Answer from the drawing. Dimensions are ordinates in mm from the lowest x, y and z of the part. A direction names the side the tool comes from. Give positions to 0.01 mm unless a question says otherwise; leave off trailing zeros. Order: outer loops, then holes, each group sorted by start corner. A loop starts at its lowest first (then second) coordinate and runs counter-clockwise, first axis right, second up.
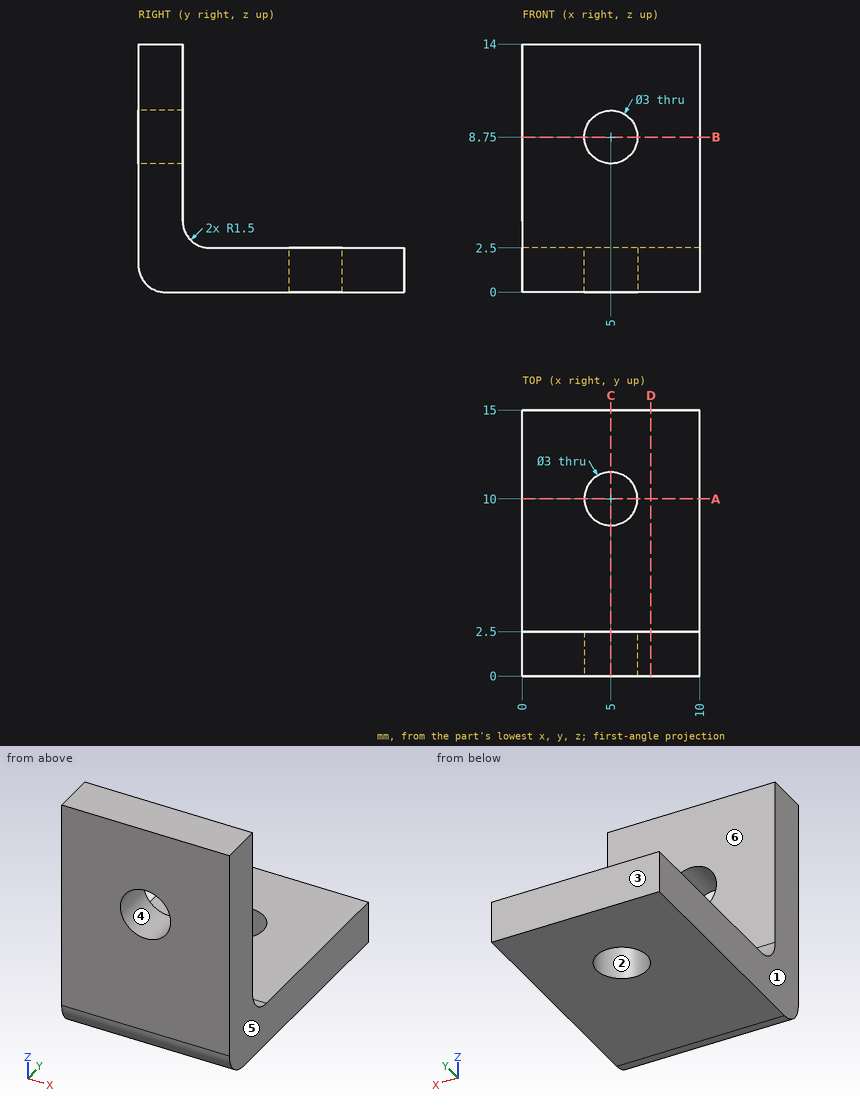
1) For a pull along X with two mould halves and no side action, classify the marked faces 1, 2, 3 and 4 as released by +X, released by -X, zero draft, split by the parting line, or undercut.
Final values:
face 1: released by -X
face 2: undercut
face 3: zero draft
face 4: undercut
2) A tool of negligible diameter and unlimited length cuts with its end or side. For the marked faces 5 and 6, from which of +Z, -Z, +X, -X, +Y, -Y can it reach the whole face along a straight path? Write none if from no direction.
Final values:
face 5: +Z, -Z, +X, +Y, -Y
face 6: +Z, +X, -X, +Y
3) The part is cut by section A-A on y = 10. Determine the outline of the cut face in (x, z).
Final values:
outline: (0, 0) - (3.5, 0) - (3.5, 2.5) - (0, 2.5) - close; (6.5, 0) - (10, 0) - (10, 2.5) - (6.5, 2.5) - close
4) The part is cut by section D-D on x = 7.25. Determine the outline of the cut face in (y, z), and give its area (4 significant figures).
Final values:
outline: (0, 1.5) arc R1.5 ccw to (1.5, 0) - (15, 0) - (15, 2.5) - (4, 2.5) arc R1.5 cw to (2.5, 4) - (2.5, 14) - (0, 14) - close
area: 66.25 mm2
5) Given pin 1 (2 mm diameter, centred on x = 3.5, y = 10, fed in from +Z); pin 2 (5 mm diameter, centred on x = 7, z = 7.5, fed in from +Y), each flat-ended and moving along its own axis, determine where each tip first touches the part or whether it passes through.
Final values:
pin 1: stops at z = 2.5
pin 2: stops at y = 2.5
6) Consider L1, parallel to X at y = 0.6, z = 8.75; L2, parallel to Y at x = 5, z = 1.95; L3, parallel to Y at x = 3, z = 4.25. Determine where each line is inside the solid, lowest interval first.
Final values:
L1: x = 0 to 3.5, 6.5 to 10
L2: y = 0 to 8.5, 11.5 to 15
L3: y = 0 to 2.5
7) The part is cut by section C-C on x = 5. Determine the outline of the cut face in (y, z), and give its area (4 significant figures).
Final values:
outline: (0, 1.5) arc R1.5 ccw to (1.5, 0) - (8.5, 0) - (8.5, 2.5) - (4, 2.5) arc R1.5 cw to (2.5, 4) - (2.5, 7.25) - (0, 7.25) - close; (0, 10.25) - (2.5, 10.25) - (2.5, 14) - (0, 14) - close; (11.5, 0) - (15, 0) - (15, 2.5) - (11.5, 2.5) - close
area: 51.25 mm2
